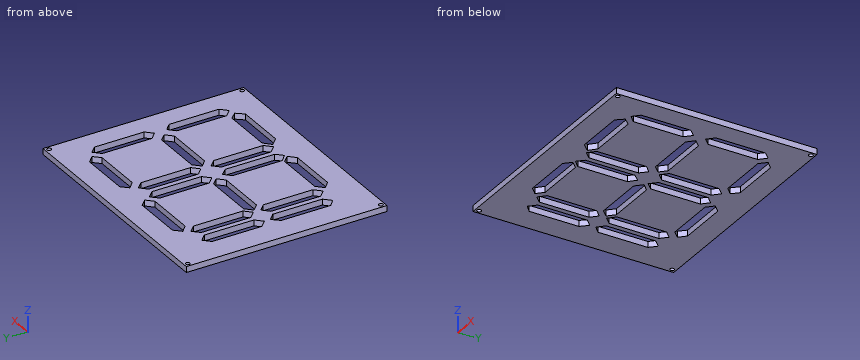
```python
from build123d import *

# Parameters (mm, degrees)
SKETCH1_W          = 201.5
SKETCH1_H          = 171.5
MAIN_BODY_DEPTH    = 5
CUT_START          = -5
CUT_AREA_OUTLINE_R = 1.8
CUT_AREA_DEPTH     = 5


# Read off the part's stored shape, not the designer's step: Cut Area
with BuildPart() as part:
    # Sketch1 → Main Body (new body)
    with BuildSketch(Plane.XY):
        Rectangle(SKETCH1_W, SKETCH1_H)
    extrude(amount=MAIN_BODY_DEPTH)

    # Cut Area outline → Cut Area (cut)
    with BuildSketch(Plane.XY.offset(5).offset(CUT_START)):
        Polygon((-68.25, 50.627106781), (-73.75, 56.127106781), (-79.25, 50.627106781), (-79.25, 8.212893219), (-73.75, 2.712893219), (-68.25, 8.212893219), align=None)
        Polygon((-73.731881274, -55.768988055), (-68.25, -50.287106781), (-68.25, -7.872893219), (-73.767236503, -2.355656716), (-79.25, -8.386696563), (-79.25, -50.802681202), align=None)
        with Locations((97.5, 82.5)):
            Circle(CUT_AREA_OUTLINE_R)
        with Locations((-97.5, -82.5)):
            Circle(CUT_AREA_OUTLINE_R)
        with Locations((97.5, -82.5)):
            Circle(CUT_AREA_OUTLINE_R)
        Polygon((-8.042893219, 6.2), (-50.457106781, 6.2), (-55.957106781, 0.7), (-50.457106781, -4.8), (-8.042893219, -4.8), (-2.542893219, 0.7), align=None)
        Polygon((-49.457106781, -55.2), (-54.957106781, -60.7), (-49.457106781, -66.2), (-7.042893219, -66.2), (-1.542893219, -60.7), (-7.042893219, -55.2), align=None)
        Polygon((5.75, 50.507106781), (0.25, 56.007106781), (-5.25, 50.507106781), (-5.25, 8.092893219), (0.25, 2.592893219), (5.75, 8.092893219), align=None)
        Polygon((0.560856139, -59.803608472), (5.75, -54.452624011), (5.75, -12.047441696), (0.561015758, -6.694204099), (-4.95, -12.036125396), (-4.95, -54.459428254), align=None)
        Polygon((66.448293895, 66.8), (24.033969108, 66.8), (18.837162213, 61.278595298), (24.657956105, 55.8), (67.072280892, 55.8), (72.269087787, 61.321404702), align=None)
        Polygon((-2.042893219, 61.3), (-7.542893219, 66.8), (-49.957106781, 66.8), (-55.457106781, 61.3), (-49.957106781, 55.8), (-7.542893219, 55.8), align=None)
        Polygon((-52.95, 8.272893219), (-52.95, 50.687106781), (-58.45, 56.187106781), (-63.95, 50.687106781), (-63.95, 8.272893219), (-58.45, 2.772893219), align=None)
        Polygon((-58.45, -56.927106781), (-52.95, -51.427106781), (-52.95, -9.012893219), (-58.45, -3.512893219), (-63.95, -9.012893219), (-63.95, -51.427106781), align=None)
        Polygon((24.042893219, 5.24), (18.542893219, -0.26), (24.042893219, -5.76), (66.457106781, -5.76), (71.957106781, -0.26), (66.457106781, 5.24), align=None)
        Polygon((83.05, 52.507106781), (77.55, 58.007106781), (72.05, 52.507106781), (72.05, 10.092893219), (77.55, 4.592893219), (83.05, 10.092893219), align=None)
        Polygon((77.55, -59.207106781), (83.05, -53.707106781), (83.05, -11.292893219), (77.55, -5.792893219), (72.05, -11.292893219), (72.05, -53.707106781), align=None)
        with Locations((-97.5, 82.5)):
            Circle(CUT_AREA_OUTLINE_R)
        Polygon((21.05, 50.507106781), (15.55, 56.007106781), (10.05, 50.507106781), (10.05, 8.092893219), (15.55, 2.592893219), (21.05, 8.092893219), align=None)
        Polygon((15.55, -59.507106781), (21.05, -54.007106781), (21.05, -11.592893219), (15.55, -6.092893219), (10.05, -11.592893219), (10.05, -54.007106781), align=None)
        Polygon((24.551704565, -55.16), (18.730025795, -60.638537988), (24.528319558, -66.8), (66.978214993, -66.8), (72.123248282, -60.640233696), (66.966029948, -55.16), align=None)
    extrude(amount=CUT_AREA_DEPTH, mode=Mode.SUBTRACT)


solid = part.part
```
Here's how the part is built. I have some questions about the finished solid (model axes, mm). Coordinates: 2 decimals unless noted, no trailing zeros. Order: outer loops, then holes, each group sorted by start corner. A loop starts at its lowest first (then second) coordinate and runs counter-clockwise, first axis right, second up.
1) Imagine slicing it at C-C on x = -34.5. List the corners of the cut face in (y, z) for me, and give its area (4 significant figures).
2) Imagine slicing it at D-D on y = 18. List the corners of the cut face in (x, z) for me, and give its area (4 significant figures).
3) Imagine slicing it at A-A on x = 53. List the corners of the cut face in (y, z) for me, and give its area (3 significant figures).
4) Imagine slicing it at B-B on y = -25. List the corners of the cut face in (x, z) for me, and give its area (3 significant figures).
5) I need wall thicknesses on line 1 (Y direction, x = 97.5, z = 3); line 2 (X direction, y = -82.5, z = 3); line 3 (X direction, y = -50, z = 2.5). Which ranges of each line are inside material? Lowest first, please.
Response values:
1. outline: (-85.75, 0) - (-66.2, 0) - (-66.2, 5) - (-85.75, 5) - close; (-55.2, 0) - (-4.8, 0) - (-4.8, 5) - (-55.2, 5) - close; (6.2, 0) - (55.8, 0) - (55.8, 5) - (6.2, 5) - close; (66.8, 0) - (85.75, 0) - (85.75, 5) - (66.8, 5) - close
1. area: 692.5 mm2
2. outline: (-100.75, 0) - (-79.25, 0) - (-79.25, 5) - (-100.75, 5) - close; (-68.25, 0) - (-63.95, 0) - (-63.95, 5) - (-68.25, 5) - close; (-52.95, 0) - (-5.25, 0) - (-5.25, 5) - (-52.95, 5) - close; (5.75, 0) - (10.05, 0) - (10.05, 5) - (5.75, 5) - close; (21.05, 0) - (72.05, 0) - (72.05, 5) - (21.05, 5) - close; (83.05, 0) - (100.75, 0) - (100.75, 5) - (83.05, 5) - close
2. area: 732.5 mm2
3. outline: (-85.75, 0) - (-66.8, 0) - (-66.8, 5) - (-85.75, 5) - close; (-55.16, 0) - (-5.76, 0) - (-5.76, 5) - (-55.16, 5) - close; (5.24, 0) - (55.8, 0) - (55.8, 5) - (5.24, 5) - close; (66.8, 0) - (85.75, 0) - (85.75, 5) - (66.8, 5) - close
3. area: 689 mm2
4. outline: (-100.75, 0) - (-79.25, 0) - (-79.25, 5) - (-100.75, 5) - close; (-68.25, 0) - (-63.95, 0) - (-63.95, 5) - (-68.25, 5) - close; (-52.95, 0) - (-4.95, 0) - (-4.95, 5) - (-52.95, 5) - close; (5.75, 0) - (10.05, 0) - (10.05, 5) - (5.75, 5) - close; (21.05, 0) - (72.05, 0) - (72.05, 5) - (21.05, 5) - close; (83.05, 0) - (100.75, 0) - (100.75, 5) - (83.05, 5) - close
4. area: 734 mm2
5. line 1: y = -85.75 to -84.3, -80.7 to 80.7, 84.3 to 85.75
5. line 2: x = -100.75 to -99.3, -95.7 to 95.7, 99.3 to 100.75
5. line 3: x = -100.75 to -79.25, -68.25 to -63.95, -52.95 to -4.95, 5.75 to 10.05, 21.05 to 72.05, 83.05 to 100.75
